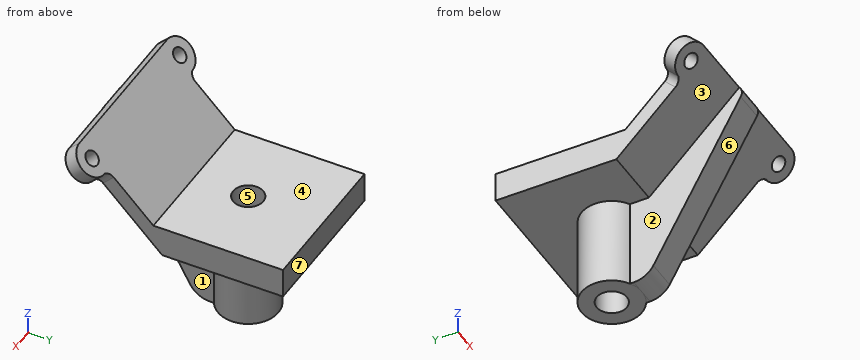
```python
from build123d import *

# Parameters (mm, degrees)
SCHIZZO1_W                   = 50
SCHIZZO1_H                   = 50
ESTRUSIONE_ESTRUSIONE1_DEPTH = 5
SCHIZZO2_R                   = 10
ESTRUSIONE_ESTRUSIONE2_DEPTH = 30
SCHIZZO3_R                   = 5
TAGLIO_ESTRUSIONE1_DEPTH     = 69.738635424
ESTRUSIONE_ESTRUSIONE6_DEPTH = 5
ESTRUSIONE_ESTRUSIONE7_REACH = 74.379
SCHIZZO9_W                   = 50
SCHIZZO9_H                   = 5
TAGLIO_ESTRUSIONE4_DEPTH     = 85.062355977
SCHIZZO12_R                  = 2.5
TAGLIO_ESTRUSIONE5_DEPTH     = 69.505418355
NERVATURA14_START            = -5
NERVATURA14_DEPTH            = 10


with BuildPart() as part:
    # Schizzo1 → Estrusione-Estrusione1 (new, symmetric)
    with BuildSketch(Plane.XY):
        with Locations((0, 25)):
            Rectangle(SCHIZZO1_W, SCHIZZO1_H)
    extrude(amount=ESTRUSIONE_ESTRUSIONE1_DEPTH, both=True)

    # Schizzo2 → Estrusione-Estrusione2 (add)
    with BuildSketch(Plane(origin=(0, 0, -5), x_dir=(-1, 0, 0), z_dir=(0, 0, -1))):
        with Locations((0, 25)):
            Circle(SCHIZZO2_R)
    extrude(amount=ESTRUSIONE_ESTRUSIONE2_DEPTH)

    # Schizzo3 → Taglio-Estrusione1 (cut, through all)
    with BuildSketch(Plane.XY.offset(5)):
        with Locations((0, 25)):
            Circle(SCHIZZO3_R)
    extrude(amount=-TAGLIO_ESTRUSIONE1_DEPTH, mode=Mode.SUBTRACT)

    # Estrusione-Estrusione7: up to this face of the body (flat: up to its plane)
    estrusione_estrusione7_end = Plane(part.part.faces().sort_by_distance((-24.292893219, 25, 5))[0])
    # Schizzo9 → Estrusione-Estrusione7 (add, up to the picked face)
    with BuildSketch(Plane(origin=(0, -2.5, 2.5), x_dir=(1, 0, 0), z_dir=(0, 0.7071067811865465, -0.7071067811865487)), mode=Mode.PRIVATE) as estrusione_estrusione7_sk1:
        with Locations((0, -6.035533906)):
            Rectangle(SCHIZZO9_W, SCHIZZO9_H)
    estrusione_estrusione7_tool1 = split(extrude(estrusione_estrusione7_sk1.sketch, amount=ESTRUSIONE_ESTRUSIONE7_REACH, mode=Mode.PRIVATE), bisect_by=estrusione_estrusione7_end, keep=Keep.BOTH, mode=Mode.PRIVATE)


with BuildPart() as body_2:
    # Schizzo4 → Estrusione-Estrusione6 (new body)
    with BuildSketch(Plane(origin=(0, 2.5, 2.5), x_dir=(1, 0, 0), z_dir=(0, 0.7071067811865488, 0.7071067811865464))):
        with BuildLine():
            ThreePointArc((-26.89463486, -19.849691999), (-32.805533406, -25.760590545), (-26.89463486, -31.67148909))
            Line((-26.89463486, -31.67148909), (0, -31.67148909))
            Line((0, -31.67148909), (0, -3.535533906))
            Line((0, -3.535533906), (-25, -3.535533906))
            Line((-25, -3.535533906), (-25, -17.060755301))
            ThreePointArc((-25, -17.060755301), (-25.518458602, -18.746564391), (-26.89463486, -19.849691999))
        make_face()
        with BuildLine():
            Line((0, -3.535533906), (0, -31.67148909))
            Line((0, -31.67148909), (26.89463486, -31.67148909))
            ThreePointArc((26.89463486, -31.67148909), (32.805533406, -25.760590545), (26.89463486, -19.849691999))
            ThreePointArc((26.89463486, -19.849691999), (25.518458602, -18.746564391), (25, -17.060755301))
            Line((25, -17.060755301), (25, -3.535533906))
            Line((25, -3.535533906), (0, -3.535533906))
        make_face()
    extrude(amount=ESTRUSIONE_ESTRUSIONE6_DEPTH)


with BuildPart() as part_1:
    add(part.part)

    add(body_2.part)  # Estrusione-Estrusione7 merges body 2
    add(estrusione_estrusione7_tool1.solids().sort_by(Axis((0, 1.767767, 6.767767), (0, 0.7071067811865465, -0.7071067811865487)))[0])

    # Schizzo11 → Taglio-Estrusione4 (cut, through all)
    with BuildSketch(Plane.ZY.offset(25)):
        Polygon((5, 0), (-5, 0), (-5, 10), align=None)
    extrude(amount=-TAGLIO_ESTRUSIONE4_DEPTH, mode=Mode.SUBTRACT)

    # Schizzo12 → Taglio-Estrusione5 (cut, through all)
    with BuildSketch(Plane(origin=(0, 6.035533906, 6.035533906), x_dir=(1, 0, 0), z_dir=(0, 0.7071067811865486, 0.7071067811865465))):
        with Locations(Location((-26.89463486, -25.760590545, 0), (0, 0, 270))):
            Circle(SCHIZZO12_R)
    taglio_estrusione5 = extrude(amount=-TAGLIO_ESTRUSIONE5_DEPTH, mode=Mode.SUBTRACT)

    # Specchia9: Taglio-Estrusione5 across plane
    add(taglio_estrusione5.mirror(Plane(origin=(0, 0, 0), x_dir=(0, 0, 1), z_dir=(1, 0, 0))), mode=Mode.SUBTRACT)

    # Nervatura14: read off the stored shape, not the designer's step
    # Nervatura14 outline → Nervatura14 (add)
    with BuildSketch(Plane(origin=(0, 0, 0), x_dir=(0, 0, -1), z_dir=(1, 0, 0)).offset(NERVATURA14_START)):
        with BuildLine():
            Line((35, 15.045679329), (34.991975911, 16.339745962))
            Line((34.991975911, 16.339745962), (5, 16.339745962))
            Line((5, 16.339745962), (5, 10))
            Line((5, 10), (-24.894153049, -19.894153049))
            ThreePointArc((-24.894153049, -19.894153049), (-23.096604523, -20.742423587), (-21.144530268, -20.368057844))
            Line((-21.144530268, -20.368057844), (31.188764864, 8.540341978))
            ThreePointArc((31.188764864, 8.540341978), (33.987865457, 11.269552189), (35, 15.045679329))
        make_face()
    extrude(amount=NERVATURA14_DEPTH)


solid = part_1.part
```
The listing builds one solid part. Answer for the finished solid, in the listing's coordinates (mm). Face numbers are marked on the shaded views. A direction names the side the tool comes from. Give positions to 0.01 mm unless a question says otherwise; leave off trailing zeros. Order: outer loops, then holes, each group sorted by start corner. A loop starts at its lowest first (then second) coordinate and runs counter-clockwise, first axis right, second up. Notation, with made-up numbers: (59.25, 45) -> (105.25, 45) arc R32 cw to (105.25, 75) -> close; hole circle Ø5 at (81, 63.25). An arc over 180 degrees is marked (long way). One line per item, written item: value.
1) Determine the mould class of the marked faces 5, 6 and 7 for opening direction Y: pulls with the +Y half, pulls with the -Y half, needs draft (parallel to the pull), parting line crosses it, or undercut.
Reported:
face 5: undercut
face 6: pulls with the -Y half
face 7: pulls with the +Y half
2) Flat-ended cylindrical pins translate along their axes: P1, Ø21.5, axis at x = -10.5, y = 19.5, coming from the +Z side; P2, Ø12, axis at x = 12.5, y = 39, coming from the -Z side; P3, Ø5, axis at x = 8.5, z = 6.5, coming from the +Y side; P4, Ø2, axis at x = -15, y = -2, coming from the -Z side. Find the tip coordinate at first contact, or state that the pin passes through.
Reported:
P1: stops at z = 5
P2: stops at z = -5
P3: stops at y = 50
P4: stops at z = 6
3) Find section D-D, the plane x = 18. Determine the outline of the cut face in (y, z), plus the area to 3 significant figures.
Reported:
outline: (-19.9, 24.9) -> (10, -5) -> (50, -5) -> (50, 5) -> (7.07, 5) -> (-16.36, 28.43) -> close
area: 603 mm^2
4) Find section C-C, the plane z = -19.5. Determine the outline of the cut face in (x, y).
Reported:
outline: (-5, 2.08) -> (5, 2.08) -> (5, 16.34) arc R10 ccw (long way) to (-5, 16.34) -> close; hole circle Ø10 at (0, 25)
5) Find section A-A, the plane y = 25. Determine the outline of the cut face in (x, z).
Reported:
outline: (-25, -5) -> (-10, -5) -> (-10, -35) -> (-5, -35) -> (-5, 5) -> (-25, 5) -> close; (5, -35) -> (10, -35) -> (10, -5) -> (25, -5) -> (25, 5) -> (5, 5) -> close
6) A tool of negligible diameter and unlimited length cuts with its end or side. For the marked faces 1, 2, 3 and 4, from which of +Z, -Z, +X, -X, +Y, -Y can it reach the whole face along a straight path? Write none if from no direction.
Reported:
face 1: -Z, +X, -Y
face 2: -Z, -X, -Y
face 3: -Z, -Y
face 4: +Z, +X, -X, +Y
7) Find the intervals of material crossed by line 1 (Z direction, x = -21, y = 16); line 2 (Y direction, x = 0, z = -15); line 3 (Y direction, x = 0, z = -11), in increasing order.
Reported:
line 1: z = -5 to 5
line 2: y = -0.4 to 20, 30 to 35
line 3: y = -2.61 to 20, 30 to 35
